Work out the finished part from the listing and answer in its coordinate system (mm). Round coordinates to 2 decimals unless told otherwise and drop trailing zeros. Order: outer loops, then holes, each group sorted by start corner. A loop starts at its lowest first (then second) coordinate and runs counter-clockwise, first axis right, second up. Notation, with made-up numbers: (86, 9) - (130, 9) arc R20 ccw to (130, 18) - close; hole circle Ø8 at (67, 26). An arc over 180 degrees is marked (long way). Use CSV: the item, a comma, the result in double quotes.
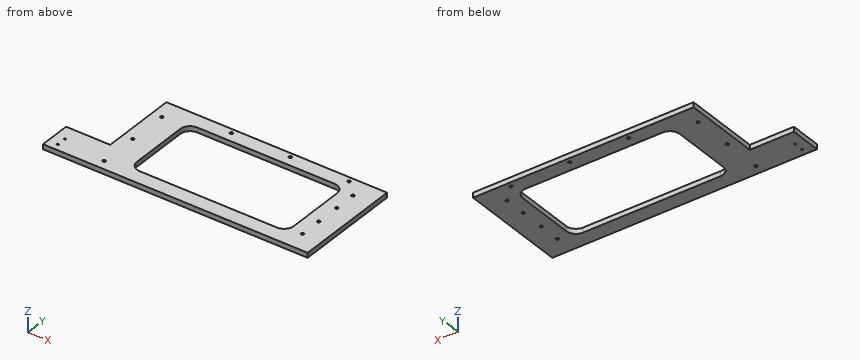
from build123d import *

# Parameters (mm, degrees)
SKETCH1_W           = 225
SKETCH1_H           = 110
BOSS_EXTRUDE1_DEPTH = 5
SKETCH2_W           = 5
SKETCH2_H           = 32
BOSS_EXTRUDE2_DEPTH = 45
SKETCH3_R           = 1.5
CUT_EXTRUDE1_DEPTH  = 6
SKETCH4_R           = 1.5
CUT_EXTRUDE2_DEPTH  = 6
SKETCH5_R           = 1
CUT_EXTRUDE3_DEPTH  = 6
SKETCH6_W           = 160
SKETCH6_H           = 80
CUT_EXTRUDE4_DEPTH  = 6
FILLET1_R           = 10


with BuildPart() as part:
    # Sketch1 → Boss-Extrude1 (new body)
    with BuildSketch(Plane.XY):
        Rectangle(SKETCH1_W, SKETCH1_H)
    extrude(amount=BOSS_EXTRUDE1_DEPTH)

    # Sketch2 → Boss-Extrude2 (add)
    with BuildSketch(Plane.ZY.offset(112.5)):
        with Locations((2.5, -39)):
            Rectangle(SKETCH2_W, SKETCH2_H)
    extrude(amount=BOSS_EXTRUDE2_DEPTH)

    # Sketch3 → Cut-Extrude1 (cut, through all)
    with BuildSketch(Plane.XY.offset(5)):
        with Locations((92.5, 35)):
            Circle(SKETCH3_R)
        with Locations((92.5, 12.5)):
            Circle(SKETCH3_R)
        with Locations((92.5, -12.5)):
            Circle(SKETCH3_R)
        with Locations((92.5, -35)):
            Circle(SKETCH3_R)
    extrude(amount=-CUT_EXTRUDE1_DEPTH, mode=Mode.SUBTRACT)

    # Sketch4 → Cut-Extrude2 (cut, through all)
    with BuildSketch(Plane.XY.offset(5)):
        with Locations((-42.5, 50)):
            Circle(SKETCH4_R)
        with Locations((-102.5, 35)):
            Circle(SKETCH4_R)
        with Locations((17.5, 50)):
            Circle(SKETCH4_R)
        with Locations((77.5, 50)):
            Circle(SKETCH4_R)
        with Locations((-102.5, -5)):
            Circle(SKETCH4_R)
        with Locations((-102.5, -45)):
            Circle(SKETCH4_R)
    extrude(amount=-CUT_EXTRUDE2_DEPTH, mode=Mode.SUBTRACT)

    # Sketch5 → Cut-Extrude3 (cut, through all)
    with BuildSketch(Plane.XY.offset(5)):
        with Locations((-147.5, -38)):
            Circle(SKETCH5_R)
        with Locations((-147.5, -48)):
            Circle(SKETCH5_R)
    extrude(amount=-CUT_EXTRUDE3_DEPTH, mode=Mode.SUBTRACT)

    # Sketch6 → Cut-Extrude4 (cut, through all)
    with BuildSketch(Plane.XY.offset(5)):
        Rectangle(SKETCH6_W, SKETCH6_H)
    extrude(amount=-CUT_EXTRUDE4_DEPTH, mode=Mode.SUBTRACT)

    # Fillet1
    fillet1_edges = [part.edges().sort_by_distance(p)[0] for p in [
        (-80, -40, 2.5),
        (-80, 40, 2.5),
        (80, 40, 2.5),
        (80, -40, 2.5),
    ]]
    fillet(fillet1_edges, radius=FILLET1_R)


solid = part.part
(1) Find the intervals of material crossed by L1, parallel to Y at x = -102.5, z = 2.05; L2, parallel to Y at x = 92.5, z = 1.7; L3, parallel to Y at x = -45.5, z = 2.6, in increasing order. Write a range as from..to.
Findings below:
L1,"y = -55..-46.5, -43.5..-6.5, -3.5..33.5, 36.5..55"
L2,"y = -55..-36.5, -33.5..-14, -11..11, 14..33.5, 36.5..55"
L3,"y = -55..-40, 40..55"
(2) Find section B-B (x = 43). Determine the outline of the cut face in (y, z).
Findings below:
outline,"(-55, 0) - (-40, 0) - (-40, 5) - (-55, 5) - close; (40, 0) - (55, 0) - (55, 5) - (40, 5) - close"
(3) This flat-tipped pin is pushed along its axis until it touches: pin 1 (2.5 mm diameter, centred on y = 18.5, z = 3.5, fed in from -X). Where does it stop, or does it pass through?
Findings below:
pin 1,"stops at x = -112.5"
(4) Find section A-A (z = 2.85). State how many separate pieces and enclosed holes the cut face has, and give its area (3 significant figures).
Findings below:
separate pieces,"1"
enclosed holes,"13"
area,"13,400 mm²"
